```python
from build123d import *


with BuildPart() as part:
    # Sketch1 → Revolve1 (revolve)
    with BuildSketch(Plane.XY, mode=Mode.PRIVATE) as revolve1_sk:
        Polygon((4, 0), (4, -12), (7.5, -12), (7.5, -9), (7.25, -9), (7.25, -7), (7.5, -7), (7.5, 0), align=None)
    revolve1 = revolve(revolve1_sk.sketch.rotate(Axis((0, -6.058624222, 0), (0, 1, 0)), 90), axis=Axis((0, -6.058624222, 0), (0, 1, 0)))

    # Mirror1: Revolve1 across plane
    add(revolve1.mirror(Plane.ZX))


solid = part.part
```
CAD build for the part. Positions are in the model's coordinates, mm. A direction names the side the tool comes from. Coordinates: 2 decimals unless noted, no trailing zeros. Write each loop counter-clockwise with the first axis right and the second up, starting at its lowest first coordinate (ties: lowest second). Pieces come first, ordered by that corner, then holes.
(1) Flat gauge pins, fed straight in: pin 1 (6 mm diameter, centred on x = 0.5, y = -2, fed in from -Z); pin 2 (6 mm diameter, centred on y = 6, z = -4, fed in from -X); pin 3 (5 mm diameter, centred on x = -4.5, y = 6.5, fed in from +Z). Where does each tip first touch, or does it go through?
(2) Cut at C-C, the plane y = -8. List the corners of the cut face in (x, z).
(3) Two-plate mould, pull along Y, no slides. Class faces 1 (the face through (3.905, 0.168, 0.867)), 2 (the face through (6.43, -7.99, -3.35)), 3 (the face through (3, 12, 3)): +Y half, -Y half, draft (parallel to the pull), parting line (faces both ways), or undercut.
(4) Drill centre lines: probe 1 along Y at (x, z) = (6.75, 2.75); probe 2 along X at (y, z) = (-3.25, 0); probe 3 along X at (y, z) = (-8.25, 2.5). Where is each one in solid material? Low to high.
(5) Cut at B-B, the plane x = 0. List the corners of the cut face in (y, z), and give its area (3 significant figures).
(6) Cut at D-D, the plane z = -5.25. List the corners of the cut face in (x, y), and give its area (3 significant figures).
(7) 3-axis set-ups, long thin cutter, end or side, ignore diameter. For faces 4 (the face through (6.43, 7.99, -3.35)), 5 (the face through (-6.324, 0.098, -4.032)): which of +Z, -Z, +X, -X, +Y, -Y reach the whole face in a straight line?
(8) Cut at A-A, the plane z = 0. List the corners of the cut face in (x, y).
Geometry says:
1. pin 1: stops at z = -7.5
1. pin 2: stops at x = -7.43
1. pin 3: stops at z = 7.23
2. outline: circle Ø14.5 at (0, 0); hole circle Ø8 at (0, 0)
3. face 1: draft
3. face 2: undercut
3. face 3: +Y half
4. probe 1: y = -12 to -9, -7 to 7, 9 to 12
4. probe 2: x = -7.5 to -4, 4 to 7.5
4. probe 3: x = -6.81 to -3.12, 3.12 to 6.81
5. outline: (-12, -7.5) - (-9, -7.5) - (-9, -7.25) - (-7, -7.25) - (-7, -7.5) - (7, -7.5) - (7, -7.25) - (9, -7.25) - (9, -7.5) - (12, -7.5) - (12, -4) - (-12, -4) - close; (-12, 4) - (12, 4) - (12, 7.5) - (9, 7.5) - (9, 7.25) - (7, 7.25) - (7, 7.5) - (-7, 7.5) - (-7, 7.25) - (-9, 7.25) - (-9, 7.5) - (-12, 7.5) - close
5. area: 166 mm2
6. outline: (-5.36, -12) - (5.36, -12) - (5.36, -9) - (5, -9) - (5, -7) - (5.36, -7) - (5.36, 7) - (5, 7) - (5, 9) - (5.36, 9) - (5.36, 12) - (-5.36, 12) - (-5.36, 9) - (-5, 9) - (-5, 7) - (-5.36, 7) - (-5.36, -7) - (-5, -7) - (-5, -9) - (-5.36, -9) - close
6. area: 254 mm2
7. face 4: none
7. face 5: +Y, -Y
8. outline: (-7.5, -12) - (-4, -12) - (-4, 12) - (-7.5, 12) - (-7.5, 9) - (-7.25, 9) - (-7.25, 7) - (-7.5, 7) - (-7.5, -7) - (-7.25, -7) - (-7.25, -9) - (-7.5, -9) - close; (4, -12) - (7.5, -12) - (7.5, -9) - (7.25, -9) - (7.25, -7) - (7.5, -7) - (7.5, 7) - (7.25, 7) - (7.25, 9) - (7.5, 9) - (7.5, 12) - (4, 12) - close
